Part model, mm, in its own coordinate system. Face numbers are marked on the shaded views. Round coordinates to 2 decimals unless told otherwise and drop trailing zeros. Loops run counter-clockwise (first coordinate to the right, second up) from the corner with the lowest first, then second, coordinate; pieces in that order, holes last. Notation, with made-up numbers: (13.25, 33.5) - (67.25, 33.5) arc R33 ccw to (67.25, 68.5) - close; hole circle Ø11 at (-15, 68). An arc over 180 degrees is marked (long way). Write each question's results on one line, items separated by ' | '. Start each with the question number.
(1) Mould opens along Z. For the marked faces 1, 2 and 3 say: released by +Z, released by -Z, zero draft, split by the parting line, or undercut.
(2) Cut at A-A, the plane z = 0.6. List the corners of the cut face in (x, y), then the cut area to 3 significant figures.
(3) Drill centre lines: L1, parallel to X at y = -3.5, z = 0.7; L2, parallel to Y at x = 7.2, z = 0.3; L3, parallel to Y at x = 7.3, z = 0.35. Where is each one in solid material? Low to high.
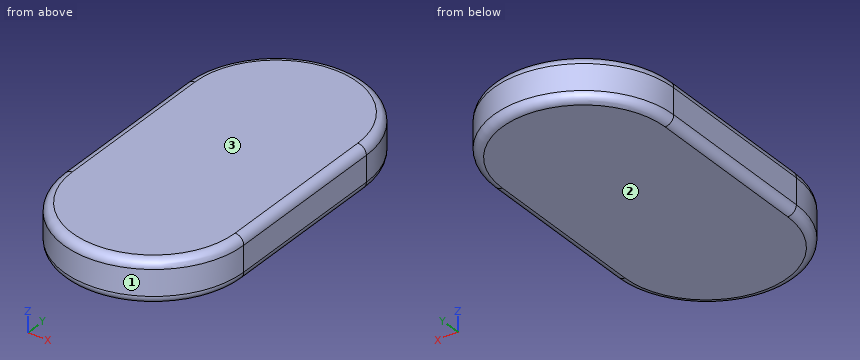
Autodesk Inventor part; units mm, degrees
ref_plane "YZ Plane" through (0, 0, 0) normal (1, 0, 0) x (0, 1, 0)
ref_plane "XZ Plane" through (0, 0, 0) normal (0, 1, 0) x (-1, 0, 0)
ref_plane "XY Plane" through (0, 0, 0) normal (0, 0, 1) x (1, 0, 0)
sketch "Skizze1" plane through (0, 0, 0) normal (0, 0, 1) x (1, 0, 0)
  arc A0 (3.65, -3.2996) -> (8.25, -3.2996) centre (5.95, -3.2996) ccw
  line L0 (8.25, 0.7004) -> (8.25, -3.2996)
  arc A1 (8.25, 0.7004) -> (3.65, 0.7004) centre (5.95, 0.7004) ccw
  line L1 (3.65, -3.2996) -> (3.65, 0.7004)
  line L2 (5.95, -3.2996) -> (5.95, 0.7004) construction
  line L3 (8.05, -3.2996) -> (8.05, 0.7004)
  line L4 (3.85, 0.7004) -> (3.85, -3.2996)
  arc A2 (3.85, -3.2996) -> (8.05, -3.2996) centre (5.95, -3.2996) ccw
  arc A3 (8.05, 0.7004) -> (3.85, 0.7004) centre (5.95, 0.7004) ccw
  point P0 (0, 0)
  point P1 (5.95, -1.2996)
  dimension "d0" = 4.2
extrude "Extrusion1" add sketch "Skizze1" along normal blind 1 contours A2 L4 A3 L3
fillet "Rundung1" radius 0.2 8 edges at (5.95, 2.8004, 1) (3.85, -1.2996, 1) (5.95, -5.3996, 1) (8.05, -1.2996, 1) (5.95, 2.8004, 0) (3.85, -1.2996, 0) (5.95, -5.3996, 0) (8.05, -1.2996, 0)
properties part number "Feets"
A:
1) face 1: zero draft | face 2: released by -Z | face 3: released by +Z
2) outline: (3.85, -3.3) arc R2.1 ccw to (8.05, -3.3) - (8.05, 0.7) arc R2.1 ccw to (3.85, 0.7) - close | area: 30.7 mm2
3) L1: 3.86 to 8.04 | L2: -4.99 to 2.39 | L3: -4.91 to 2.31
